Source: CAD feature listing. Evaluate the final solid. Frame: model axes, mm. A direction names the side the tool comes from. Give positions to 0.01 mm unless a question says otherwise; leave off trailing zeros. Order: outer loops, then holes, each group sorted by start corner. A loop starts at its lowest first (then second) coordinate and runs counter-clockwise, first axis right, second up.
Autodesk Fusion 360 part; units mm, degrees
sketch "Sketch1" plane through (0, 0, 0) normal (0, 1, 0) x (1, 0, 0)
  line L0 (-4.4022, -9.8222) -> (-3.1214, -8.5414)
  arc A0 (10, -4.8314) -> (9.8222, -4.4022) centre (9.3929, -4.8314) ccw
  line L1 (6.5607, -5.5) -> (3.9, -2.8393)
  line L2 (-9.9987, -4.7917) -> (-10, -9.5)
  line L3 (9.8222, -4.4022) -> (8.5414, -3.1214)
  arc A1 (-3.2628, 8.2) -> (-3.1214, 8.5414) centre (-3.2628, 8.4) ccw
  line L4 (3.9, 2.8393) -> (6.5607, 5.5)
  arc A2 (-8.5414, 3.1214) -> (-8.2, 3.2628) centre (-8.4, 3.2628) ccw
  line L5 (-4.8314, 10) -> (-9.5, 10)
  line L6 (-6.5607, 5.5) -> (-3.9, 2.8393)
  arc A3 (-9.5, 10) -> (-10, 9.5) centre (-9.5, 9.5) ccw
  arc A4 (8.2, 3.2628) -> (8.5414, 3.1214) centre (8.4, 3.2628) ccw
  line L7 (-5.5, 6.5607) -> (-5.5, 8.2)
  line L8 (6.5607, 5.5) -> (8.2, 5.5)
  line L9 (8.5414, 3.1214) -> (9.8222, 4.4022)
  arc A5 (3.1214, 8.5414) -> (3.2628, 8.2) centre (3.2628, 8.4) ccw
  line L10 (-8.2, 3.2628) -> (-8.2, 5.5)
  line L11 (9.5, 10) -> (4.8314, 10)
  arc A6 (10, 9.5) -> (9.5, 10) centre (9.5, 9.5) ccw
  line L12 (10, 4.8314) -> (10, 9.5)
  arc A7 (-4.4312, 9.8494) -> (-4.8314, 10) centre (-4.8314, 9.3929) ccw
  line L13 (-9.8494, 4.4312) -> (-8.5414, 3.1214)
  line L14 (4.4022, 9.8222) -> (3.1214, 8.5414)
  line L15 (-5.5, 8.2) -> (-3.2628, 8.2)
  line L16 (5.5, 8.2) -> (5.5, 6.5607)
  arc A8 (-10, 4.9) -> (-9.8494, 4.4312) centre (-9.3734, 4.8428) ccw
  circle A9 centre (0, 0) radius 2.1
  arc A10 (4.8314, 10) -> (4.4022, 9.8222) centre (4.8314, 9.3929) ccw
  line L17 (-2.8393, 3.9) -> (-5.5, 6.5607)
  line L18 (5.5, 6.5607) -> (2.8393, 3.9)
  line L19 (-3.9, 2.8393) -> (-3.9, -2.8393)
  line L20 (-10, 9.5) -> (-10, 4.9)
  line L21 (2.8393, 3.9) -> (-2.8393, 3.9)
  line L22 (3.9, -2.8393) -> (3.9, 2.8393)
  line L23 (3.2628, 8.2) -> (5.5, 8.2)
  line L24 (8.2, 5.5) -> (8.2, 3.2628)
  line L25 (5.5, -6.5607) -> (5.5, -8.2)
  arc A11 (4.2336, -9.6536) -> (4.8314, -10) centre (4.8837, -9.2207) ccw
  arc A12 (-4.8314, -10) -> (-4.4022, -9.8222) centre (-4.8314, -9.3929) ccw
  line L26 (-5.5, -6.5607) -> (-2.8393, -3.9)
  line L27 (10, -9.5) -> (10, -4.8314)
  line L28 (-8.5414, -3.1214) -> (-9.8222, -4.4022)
  line L29 (5.5, -8.2) -> (3.2628, -8.2)
  line L30 (4.8314, -10) -> (9.5, -10)
  line L31 (-8.2, -5.5) -> (-8.2, -3.2628)
  arc A13 (8.5414, -3.1214) -> (8.2, -3.2628) centre (8.4, -3.2628) ccw
  line L32 (-2.8393, -3.9) -> (2.8393, -3.9)
  arc A14 (-8.2, -3.2628) -> (-8.5414, -3.1214) centre (-8.4, -3.2628) ccw
  arc A15 (-3.1214, -8.5414) -> (-3.2628, -8.2) centre (-3.2628, -8.4) ccw
  line L33 (3.1214, -8.5414) -> (4.2336, -9.6536)
  line L34 (-5.5, -8.2) -> (-5.5, -6.5607)
  line L35 (-6.5607, -5.5) -> (-8.2, -5.5)
  line L36 (8.2, -3.2628) -> (8.2, -5.5)
  arc A16 (-9.8222, -4.4022) -> (-9.9987, -4.7917) centre (-9.3929, -4.8314) ccw
  line L37 (-9.5, -10) -> (-4.8314, -10)
  arc A17 (-10, -9.5) -> (-9.5, -10) centre (-9.5, -9.5) ccw
  arc A18 (3.2628, -8.2) -> (3.1214, -8.5414) centre (3.2628, -8.4) ccw
  line L38 (8.2, -5.5) -> (6.5607, -5.5)
  line L39 (-3.2628, -8.2) -> (-5.5, -8.2)
  line L40 (-3.9, -2.8393) -> (-6.5607, -5.5)
  line L41 (2.8393, -3.9) -> (5.5, -6.5607)
  arc A19 (9.5, -10) -> (10, -9.5) centre (9.5, -9.5) ccw
  line L42 (-3.1214, 8.5414) -> (-4.4312, 9.8494)
  arc A20 (9.8222, 4.4022) -> (10, 4.8314) centre (9.3929, 4.8314) ccw
  line L43 (-8.2, 5.5) -> (-6.5607, 5.5)
  line L44 (4, 2.7979) -> (6.6021, 5.4)
  line L45 (6.6021, 5.4) -> (8.1, 5.4)
  line L46 (8.1, 5.4) -> (8.1, 3.2628)
  arc A21 (8.1, 3.2628) -> (8.6121, 3.0507) centre (8.4, 3.2628) ccw
  line L47 (8.6121, 3.0507) -> (9.8929, 4.3315)
  arc A22 (9.8929, 4.3315) -> (10.1, 4.8314) centre (9.3929, 4.8314) ccw
  line L48 (10.1, 4.8314) -> (10.1, 9.5)
  arc A23 (10.1, 9.5) -> (9.5, 10.1) centre (9.5, 9.5) ccw
  line L49 (9.5, 10.1) -> (4.8314, 10.1)
  arc A24 (4.8314, 10.1) -> (4.3315, 9.8929) centre (4.8314, 9.3929) ccw
  line L50 (4.3315, 9.8929) -> (3.0507, 8.6121)
  arc A25 (3.0507, 8.6121) -> (3.2628, 8.1) centre (3.2628, 8.4) ccw
  line L51 (3.2628, 8.1) -> (5.4, 8.1)
  line L52 (5.4, 8.1) -> (5.4, 6.6021)
  line L53 (5.4, 6.6021) -> (2.7979, 4)
  line L54 (2.7979, 4) -> (-2.7979, 4)
  line L55 (-2.7979, 4) -> (-5.4, 6.6021)
  line L56 (-5.4, 6.6021) -> (-5.4, 8.1)
  line L57 (-5.4, 8.1) -> (-3.2628, 8.1)
  arc A26 (-3.2628, 8.1) -> (-3.0509, 8.6124) centre (-3.2628, 8.4) ccw
  line L58 (-3.0509, 8.6124) -> (-4.3627, 9.9223)
  arc A27 (-4.3627, 9.9223) -> (-4.8314, 10.1) centre (-4.8314, 9.3929) ccw
  line L59 (-4.8314, 10.1) -> (-9.5, 10.1)
  arc A28 (-9.5, 10.1) -> (-10.1, 9.5) centre (-9.5, 9.5) ccw
  line L60 (-10.1, 9.5) -> (-10.1, 4.9044)
  arc A29 (-10.1, 4.9044) -> (-9.9226, 4.363) centre (-9.3734, 4.8428) ccw
  line L61 (-9.9226, 4.363) -> (-8.6124, 3.0509)
  arc A30 (-8.6124, 3.0509) -> (-8.1, 3.2628) centre (-8.4, 3.2628) ccw
  line L62 (-8.1, 3.2628) -> (-8.1, 5.4)
  line L63 (-8.1, 5.4) -> (-6.6021, 5.4)
  line L64 (-6.6021, 5.4) -> (-4, 2.7979)
  line L65 (-4, 2.7979) -> (-4, -2.7979)
  line L66 (-4, -2.7979) -> (-6.6021, -5.4)
  line L67 (-6.6021, -5.4) -> (-8.1, -5.4)
  line L68 (-8.1, -5.4) -> (-8.1, -3.2628)
  arc A31 (-8.1, -3.2628) -> (-8.6121, -3.0507) centre (-8.4, -3.2628) ccw
  line L69 (-8.6121, -3.0507) -> (-9.8929, -4.3315)
  arc A32 (-9.8929, -4.3315) -> (-10.0987, -4.7886) centre (-9.3929, -4.8314) ccw
  line L70 (-10.0987, -4.7886) -> (-10.1, -9.4997)
  arc A33 (-10.1, -9.4997) -> (-9.5, -10.1) centre (-9.5, -9.5) ccw
  line L71 (-9.5, -10.1) -> (-4.8314, -10.1)
  arc A34 (-4.8314, -10.1) -> (-4.3315, -9.8929) centre (-4.8314, -9.3929) ccw
  line L72 (-4.3315, -9.8929) -> (-3.0507, -8.6121)
  arc A35 (-3.0507, -8.6121) -> (-3.2628, -8.1) centre (-3.2628, -8.4) ccw
  line L73 (-3.2628, -8.1) -> (-5.4, -8.1)
  line L74 (-5.4, -8.1) -> (-5.4, -6.6021)
  line L75 (-5.4, -6.6021) -> (-2.7979, -4)
  line L76 (-2.7979, -4) -> (2.7979, -4)
  line L77 (2.7979, -4) -> (5.4, -6.6021)
  line L78 (5.4, -6.6021) -> (5.4, -8.1)
  line L79 (5.4, -8.1) -> (3.2628, -8.1)
  arc A36 (3.2628, -8.1) -> (3.0507, -8.6121) centre (3.2628, -8.4) ccw
  line L80 (3.0507, -8.6121) -> (4.1561, -9.7175)
  arc A37 (4.1561, -9.7175) -> (4.8282, -10.1) centre (4.8837, -9.2207) ccw
  line L81 (4.8282, -10.1) -> (9.5, -10.1)
  arc A38 (9.5, -10.1) -> (10.1, -9.5) centre (9.5, -9.5) ccw
  line L82 (10.1, -9.5) -> (10.1, -4.8314)
  arc A39 (10.1, -4.8314) -> (9.8929, -4.3315) centre (9.3929, -4.8314) ccw
  line L83 (9.8929, -4.3315) -> (8.6121, -3.0507)
  arc A40 (8.6121, -3.0507) -> (8.1, -3.2628) centre (8.4, -3.2628) ccw
  line L84 (8.1, -3.2628) -> (8.1, -5.4)
  line L85 (8.1, -5.4) -> (6.6021, -5.4)
  line L86 (6.6021, -5.4) -> (4, -2.7979)
  line L87 (4, -2.7979) -> (4, 2.7979)
  line L88 (9, 9) -> (25.1, 9)
  line L89 (25.1, 9) -> (25.1, -17)
  line L90 (25.1, -17) -> (9, -17)
  line L91 (9, -17) -> (9, 9)
  line L92 (10.1, -5.988) -> (10.1, -17)
  dimension "d1" = 0.1
  dimension "d2" = 16.1
  dimension "d3" = 26
extrude "Extrude1" add sketch "Sketch1" along normal blind 25 contours L47 A22 L48 L82 A39 L83 L88 L89 L90 L91 L92 | L44 L45 L46 A21 L47 L83 A40 L84 L85 L86 L87 L91
fillet "Fillet1" radius 15 1 edges at (25.1, 12.5, -9)
sketch "Sketch2" plane through (0, 0, 17) normal (0, 0, 1) x (-1, 0, 0)
  line L0 (-10.1, 0) -> (-25.1, 0)
  line L1 (-25.1, 0) -> (-25.1, -25)
  line L2 (-25.1, -25) -> (-10.1, -25)
  line L3 (-10.1, -25) -> (-10.1, 0)
  line L4 (-10.1, 0) -> (-12.1, 0) construction
  line L5 (-12.1, 0) -> (-25.1, 0) construction
  line L6 (-18.6, 0) -> (-18.6, -25) construction
  line L7 (-25.1, -12.5) -> (-18.6, -12.5) construction
  line L8 (-25.1, -2.55) -> (-12.1, -2.55)
  line L9 (-12.1, -2.55) -> (-12.1, -22.45)
  line L10 (-12.1, -22.45) -> (-25.1, -22.45)
  line L11 (-25.1, -22.45) -> (-25.1, -2.55)
  line L12 (-25.1, -2.55) -> (-12.1, -22.45) construction
  line L13 (-12.1, -2.55) -> (-25.1, -22.45) construction
  line L14 (-12.1, -2.55) -> (-19.8, -2.55) construction
  line L15 (-19.8, -2.55) -> (-19.8, -22.45) construction
  line L16 (-19.8, -2.55) -> (-19.8, -7.7) construction
  line L17 (-19.8, -7.7) -> (-19.8, -17.3) construction
  line L18 (-19.8, -17.3) -> (-19.8, -22.45) construction
  circle A0 centre (-19.8, -7.7) radius 1.05
  circle A1 centre (-19.8, -17.3) radius 1.05
  line L19 (-12.1, -2.55) -> (-10.1, -2.55)
  line L20 (-10.1, -2.55) -> (-10.1, -22.45)
  line L21 (-10.1, -22.45) -> (-12.1, -22.45)
  line L22 (-12.1, -22.45) -> (-12.1, -2.55)
  point P0 (-18.6, -12.5)
  dimension "d8" = 2
  dimension "d9" = 19.9
  dimension "d10" = 7.7
  dimension "d11" = 5.15
  dimension "d12" = 9.6
  dimension "d13" = 5.15
  dimension "d14" = 2.1
  dimension "d15" = 2.1
  dimension "d16" = 19.9
extrude "Extrude2" cut sketch "Sketch2" against normal blind 6.5 contours L3 L9 L19 L20 L21 L22 | L1 L8 L9 L10 L11 L22
sketch "Sketch3" plane through (0, 25, 0) normal (0, 1, 0) x (-1, 0, 0)
  arc A0 (-25.1, 6) -> (-10.1, -9) centre (-10.1, 6) ccw
  line L0 (-10.1, -9) -> (-10.1, -4.8314)
  arc A1 (-9.8929, -4.3315) -> (-10.1, -4.8314) centre (-9.3929, -4.8314) ccw
  line L1 (-9.8929, -4.3315) -> (-8.6121, -3.0507)
  arc A2 (-8.1, -3.2628) -> (-8.6121, -3.0507) centre (-8.4, -3.2628) ccw
  line L2 (-8.1, -3.2628) -> (-8.1, -5.4)
  line L3 (-8.1, -5.4) -> (-6.6021, -5.4)
  line L4 (-6.6021, -5.4) -> (-4, -2.7979)
  line L5 (-4, -2.7979) -> (-4, 2.7979)
  line L6 (-4, 2.7979) -> (-6.6021, 5.4)
  line L7 (-6.6021, 5.4) -> (-8.1, 5.4)
  line L8 (-8.1, 5.4) -> (-8.1, 3.2628)
  arc A3 (-8.6121, 3.0507) -> (-8.1, 3.2628) centre (-8.4, 3.2628) ccw
  line L9 (-8.6121, 3.0507) -> (-9.8929, 4.3315)
  arc A4 (-10.1, 4.8314) -> (-9.8929, 4.3315) centre (-9.3929, 4.8314) ccw
  line L10 (-10.1, 4.8314) -> (-10.1, 5.988)
  line L11 (-10.1, 5.988) -> (-10.1, 17)
  line L12 (-10.1, 17) -> (-25.1, 17)
  line L13 (-25.1, 17) -> (-25.1, 6)
  line L14 (-12.95, 2.8) -> (-11.05, 2.8)
  line L15 (-11.05, 2.8) -> (-11.05, -2.8)
  line L16 (-11.05, -2.8) -> (-12.95, -2.8)
  line L17 (-12.95, -2.8) -> (-12.95, 2.8)
  line L18 (-12.95, 2.8) -> (-11.05, -2.8) construction
  line L19 (-11.05, 2.8) -> (-12.95, -2.8) construction
  point P0 (-12, 0)
  dimension "d19" = 1.9
  dimension "d20" = 5.6
sketch "Sketch4" plane through (4, 0, 0) normal (-1, 0, 0) x (0, -1, 0)
  line L0 (0, -2.7979) -> (0, 2.7979)
  line L1 (0, 2.7979) -> (-25, 2.7979)
  line L2 (-25, 2.7979) -> (-25, -2.7979)
  line L3 (-25, -2.7979) -> (0, -2.7979)
  line L4 (0, 0) -> (-12.5, 0) construction
  circle A0 centre (-12.5, 0) radius 1.55
  circle A1 centre (-12.5, 0) radius 3
  dimension "d21" = 3.1
  dimension "d22" = 6
extrude "Extrude3" cut sketch "Sketch4" against normal blind 21 contours A0
extrude "Extrude4" cut sketch "Sketch4" against normal blind 10 from surface at -12 contours L3 A1 | L1 L3 A1 | L1 A1
extrude "Extrude5" cut sketch "Sketch3" along normal blind 15.5 from surface at -25 contours L14 L15 L16 L17
1) Section query A-A, the plane z = 11. Return the cut outline in (x, y).
Report:
outline: (10.1, 0) - (25.1, 0) - (25.1, 2.55) - (10.1, 2.55) - close; (10.1, 22.45) - (25.1, 22.45) - (25.1, 25) - (10.1, 25) - close; circle Ø2.1 at (19.8, 7.7); circle Ø2.1 at (19.8, 17.3)
2) Material intervals for L1, parallel to Y at x = 13.25, z = 12.5; L2, parallel to Y at x = 22.75, z = 0; L3, parallel to Z at x = 5.75, y = 12.5, sorted ascending.
Report:
L1: y = 0 to 2.55, 22.45 to 25
L2: y = 0 to 9.5, 15.5 to 25
L3: z = -4.55 to -1.55, 1.55 to 4.55
3) Reachability of faces 1 (the flat face through (7, 12, 5.4)), 2 (the flat face through (8.1, 12, 4)), 3 (the flat face through (8.1, 12, -4)), 4 (the flat face through (18, 2.55, 14)) from +Z, -Z, +X, -X, +Y, -Y: full face, straight path, thin tool, end or side. Return the list, or none.
Report:
face 1: +Z, -X, +Y, -Y
face 2: +Z, +Y, -Y
face 3: -Z, +Y, -Y
face 4: +Z, +X, -X
4) Section query C-C, the plane x = 19.25. Return the cut outline in (y, z).
Report:
outline: (0, -5.89) - (25, -5.89) - (25, 17) - (22.45, 17) - (22.45, 10.5) - (18.19, 10.5) - (18.19, 17) - (16.41, 17) - (16.41, 10.5) - (8.59, 10.5) - (8.59, 17) - (6.81, 17) - (6.81, 10.5) - (2.55, 10.5) - (2.55, 17) - (0, 17) - close; hole circle Ø6 at (12.5, 0)
5) Pin query (flat end, axial travel): pin 1 (3 mm diameter, centred on x = 8.5, y = 21.5, fed in from -Z); pin 2 (1.5 mm diameter, centred on x = 12, y = 9, fed in from +Z); pin 3 (1 mm diameter, centred on x = 11.5, z = 3.5, fed in from -Y); pin 4 (1.7 mm diameter, centred on y = 7, z = 0, fed in from +X). Return the tip coordinate at first contact, or that it passes through.
Report:
pin 1: stops at z = -5.4
pin 2: stops at z = 10.5
pin 3: stops at y = 0
pin 4: stops at x = 24.19
6) Draft query along Z for faces 5 (the flat face through (18, 1, 17)), 6 (the flat face through (17, 0, 4)), 7 (the flat face through (12, 8, 2.8)). Return one class per face: +Z half, -Z half, draft (parallel to the pull), parting line (faces both ways), or undercut.
Report:
face 5: +Z half
face 6: draft
face 7: undercut
7) Section query D-D, the plane z = 0. Return the cut outline in (x, y), and give its area (3 significant figures).
Report:
outline: (4, 0) - (11.05, 0) - (11.05, 10.95) - (4, 10.95) - close; (4, 14.05) - (11.05, 14.05) - (11.05, 15.5) - (12.95, 15.5) - (12.95, 14.05) - (16, 14.05) - (16, 15.5) - (23.85, 15.5) - (23.85, 25) - (4, 25) - close; (12.95, 0) - (23.85, 0) - (23.85, 9.5) - (16, 9.5) - (16, 10.95) - (12.95, 10.95) - close
area: 388 mm2
